Work out the finished part from the listing and answer in its coordinate system (mm). A direction names the side the tool comes from. Round coordinates to 2 decimals unless told otherwise and drop trailing zeros. Order: outer loops, then holes, each group sorted by start corner. A loop starts at its lowest first (then second) coordinate and runs counter-clockwise, first axis right, second up. Notation, with made-up numbers: (59, 71) - (100, 71) arc R24 ccw to (100, 86) - close; hole circle Ø9 at (49, -35). An arc over 180 degrees is marked (long way). Use one line per item in the form item = value. Start each with the question number.
Q1. For a pull along Y with two mould halves and no side action, classify faces 1 (the flat face through (32.5, 20, 0)), 2 (the cylindrical face through (-29.49, 42.15, 0.14)), 3 (the flat face through (20.25, 24, 6)) as +Y half, -Y half, draft (parallel to the pull), parting line (faces both ways), or undercut.
Q2. The part is cut by section C-C on y = 25. Determine the outline of the cut face in (x, z).
Q3. The part is cut by section A-A on x = 13. Determine the outline of the cut face in (y, z).
Q4. Which of the six approach directions +Z, -Z, +X, -X, +Y, -Y give full straight-line access (tool end or side, diameter ignored) to faces 4 (the flat face through (-40, 5, 0)), 5 (the flat face through (0, 19.9, 0)), 6 (the flat face through (-22, 32.5, 6))?
Q5. Find the intervals of material crossed by line 1 (X direction, y = 3.8, z = 0); line 2 (Y direction, x = -18, z = 6.25); line 3 (X direction, y = 23, z = 8), in increasing order. Write a range as [from, to].
Q6. The part is cut by section D-D on x = -24.15. Determine the outline of the cut face in (y, z).
Q7. Given P1, Ø5, axis at y = 12, z = 3, coming from the -X side; P2, Ø10, axis at y = 24.5, z = 0, coming from the +X side; P3, Ø3, axis at y = 38, z = 3, coming from the +X side; P4, Ø4, axis at x = 25, z = -1.5, coming from the -Y side, each flat-ended and moving along its own axis, determine where each tip first touches the part or whether it passes through.
Q8. The part is cut by section B-B on z = 0. Determine the outline of the cut face in (x, y).
from build123d import *

# Parameters (mm, degrees)
BOSS_EXTRUDE1_DEPTH = 10
SKETCH3_R           = 1.55
CUT_EXTRUDE1_DEPTH  = 12
SKETCH3_3_R         = 1.55
SKETCH3_3_W         = 3
SKETCH3_3_H         = 5
CUT_EXTRUDE3_DEPTH  = 21
SKETCH5_R           = 1.55
CUT_EXTRUDE4_DEPTH  = 6
FILLET1_R           = 1


with BuildPart() as part:
    # Sketch1 → Boss-Extrude1 (new body, symmetric)
    with BuildSketch(Plane.XY):
        with BuildLine():
            Line((-42.5, 0), (42.5, 0))
            Line((42.5, 0), (42.5, 5))
            Line((42.5, 5), (32.5, 5))
            Line((32.5, 5), (32.5, 35))
            ThreePointArc((32.5, 35), (29.571067812, 42.071067812), (22.5, 45))
            Line((22.5, 45), (-22.5, 45))
            ThreePointArc((-22.5, 45), (-29.571067812, 42.071067812), (-32.5, 35))
            Line((-32.5, 35), (-32.5, 5))
            Line((-32.5, 5), (-42.5, 5))
            Line((-42.5, 5), (-42.5, 0))
        make_face()
    extrude(amount=BOSS_EXTRUDE1_DEPTH, both=True)

    # Sketch3 → Cut-Extrude1 (cut)
    with BuildSketch(Plane(origin=(0, 0, -10), x_dir=(-1, 0, 0), z_dir=(0, 0, -1))):
        Polygon((-27.6, 40.1), (-27.6, 19.9), (-20.25, 19.9), (-20.25, 27.5), (-23.25, 27.5), (-23.25, 32.5), (-20.25, 32.5), (-20.25, 40.1), align=None)
        with Locations((-24.15, 25)):
            Circle(SKETCH3_R, mode=Mode.SUBTRACT)
        with Locations((-24.15, 35)):
            Circle(SKETCH3_R, mode=Mode.SUBTRACT)
        Polygon((20.25, 27.5), (20.25, 19.9), (27.6, 19.9), (27.6, 40.1), (20.25, 40.1), (20.25, 32.5), (23.25, 32.5), (23.25, 27.5), align=None)
        with Locations((24.15, 25)):
            Circle(SKETCH3_R, mode=Mode.SUBTRACT)
        with Locations((24.15, 35)):
            Circle(SKETCH3_R, mode=Mode.SUBTRACT)
    extrude(amount=-CUT_EXTRUDE1_DEPTH, mode=Mode.SUBTRACT)

    # Sketch3_3 → Cut-Extrude3 (cut, through all)
    with BuildSketch(Plane(origin=(0, 0, -10), x_dir=(-1, 0, 0), z_dir=(0, 0, -1))):
        Polygon((-20.25, 27.5), (-20.25, 19.9), (20.25, 19.9), (20.25, 27.5), (20.25, 32.5), (20.25, 40.1), (-20.25, 40.1), (-20.25, 32.5), align=None)
        with Locations((-24.15, 25)):
            Circle(SKETCH3_3_R)
        with Locations((24.15, 35)):
            Circle(SKETCH3_3_R)
        with Locations((-21.75, 30)):
            Rectangle(SKETCH3_3_W, SKETCH3_3_H)
        with Locations((21.75, 30)):
            Rectangle(SKETCH3_3_W, SKETCH3_3_H)
        with Locations((-24.15, 35)):
            Circle(SKETCH3_3_R)
        with Locations((24.15, 25)):
            Circle(SKETCH3_3_R)
    extrude(amount=-CUT_EXTRUDE3_DEPTH, mode=Mode.SUBTRACT)

    # Sketch5 → Cut-Extrude4 (cut, through all)
    with BuildSketch(Plane(origin=(0, 5, 0), x_dir=(1, 0, 0), z_dir=(0, 1, 0))):
        with Locations((37.5, 0)):
            Circle(SKETCH5_R)
    cut_extrude4 = extrude(amount=-CUT_EXTRUDE4_DEPTH, mode=Mode.SUBTRACT)

    # Mirror3: Cut-Extrude4 across plane
    add(cut_extrude4.mirror(Plane(origin=(0, 0, 0), x_dir=(0, 0, 1), z_dir=(1, 0, 0))), mode=Mode.SUBTRACT)

    # Fillet1
    fillet1_edges = [part.edges().sort_by_distance(p)[0] for p in [
        (-42.5, 2.5, -10),
        (42.5, 2.5, -10),
        (-32.5, 5, 0),
        (32.5, 5, 0),
        (-42.5, 2.5, 10),
        (42.5, 2.5, 10),
    ]]
    fillet(fillet1_edges, radius=FILLET1_R)


solid = part.part
Found:
q1.face_1 = draft
q1.face_2 = +Y half
q1.face_3 = undercut
q2.outline = (-32.5, -10) - (-27.6, -10) - (-27.6, 2) - (-25.7, 2) - (-25.7, 10) - (-32.5, 10) - close; (-22.6, 2) - (-20.25, 2) - (-20.25, 10) - (-22.6, 10) - close; (20.25, 2) - (22.6, 2) - (22.6, 10) - (20.25, 10) - close; (25.7, 2) - (27.6, 2) - (27.6, -10) - (32.5, -10) - (32.5, 10) - (25.7, 10) - close
q3.outline = (0, -10) - (19.9, -10) - (19.9, 10) - (0, 10) - close; (40.1, -10) - (45, -10) - (45, 10) - (40.1, 10) - close
q4.face_4 = +Z, -Z, -X, +Y
q4.face_5 = -Z
q4.face_6 = +Z, -Z
q5.line_1 = [-42.5, -39.05], [-35.95, 35.95], [39.05, 42.5]
q5.line_2 = [0, 19.9], [40.1, 45]
q5.line_3 = [-32.5, -20.25], [20.25, 32.5]
q6.outline = (0, -10) - (19.9, -10) - (19.9, 2) - (23.45, 2) - (23.45, 10) - (0, 10) - close; (26.55, 2) - (33.45, 2) - (33.45, 10) - (26.55, 10) - close; (36.55, 2) - (40.1, 2) - (40.1, -10) - (44.86, -10) - (44.86, 10) - (36.55, 10) - close
q7.P1 = -32.5
q7.P2 = 32.5
q7.P3 = 32.39
q7.P4 = 0
q8.outline = (-42.5, 0) - (-39.05, 0) - (-39.05, 5) - (-42.5, 5) - close; (-35.95, 0) - (35.95, 0) - (35.95, 5) - (33.5, 5) arc R1 cw to (32.5, 6) - (32.5, 35) arc R10 ccw to (22.5, 45) - (-22.5, 45) arc R10 ccw to (-32.5, 35) - (-32.5, 6) arc R1 cw to (-33.5, 5) - (-35.95, 5) - close; (39.05, 0) - (42.5, 0) - (42.5, 5) - (39.05, 5) - close; hole (-27.6, 19.9) - (27.6, 19.9) - (27.6, 40.1) - (-27.6, 40.1) - close
